Source: CAD feature listing. Evaluate the final solid. Frame: model axes, mm. A direction names the side the tool comes from. Coordinates: 2 decimals unless noted, no trailing zeros. Order: outer loops, then holes, each group sorted by start corner. A loop starts at its lowest first (then second) coordinate and runs counter-clockwise, first axis right, second up. Notation, with made-up numbers: (8, -13) -> (67, -13) arc R16 cw to (67, -2) -> close; hole circle Ø9 at (74.25, -17). An arc over 180 degrees is marked (long way). Write item = value, one per line. Start each with the question number.
Item 1: Section query C-C (y = 9). Output: boundary loops of the cut face in (x, z).
Item 2: Contact query for flat-ended pins moving along their axis: pin 1 (2 mm diameter, centred on x = 24.5, y = -39, fed in from +Z); pin 2 (5 mm diameter, centred on x = 26, z = -12.5, fed in from -Y); pin 3 (12 mm diameter, centred on y = 19.5, z = -18, fed in from -X). Output: stop coordinate, or through.
Item 3: Ray query, line 1 along Z through (x, y) = (16.25, 26.5); line 2 along Y through (x, z) = (28.75, -15); line 3 along Y through (x, z) = (21.75, -2). Return the intervals inside material, ascending. Write a range as [from, to].
Item 4: Mould query, pull axis Z, two halves, no side actions, for faces 4 (the flat face through (26.737, 26, 0)), 5 (the flat face through (26, 23, -2.473)), 6 (the flat face through (25.094, -47.195, 0.467)), 7 (the flat face through (25.02, -47.19, 1.6)). Classes: released by +Z, released by -Z, zero draft, split by the parting line, or undercut.
Item 5: Set-up query: faces 1 (the flat face through (28.04, -47.19, 1.47)), 2 (the flat face through (26.54, -47.34, -10.64)), 3 (the flat face through (26, 23, 2.253)). Return all of +Z, -Z, +X, -X, +Y, -Y with unobstructed straight access to the full face (end or side cutting, diameter ignored); none if empty.
Item 6: Section query B-B (z = 21). Output: boundary loops of the cut face in (x, y), then the cut area to 3 significant figures.
Item 7: Section query D-D (x = 30). Output: boundary loops of the cut face in (y, z), then the cut area to 3 significant figures.
Item 8: Section query A-A (z = -14.5). Output: boundary loops of the cut face in (x, y), then the cut area to 3 significant figures.
```python
from build123d import *

# Parameters (mm, degrees)
BOSS_EXTRUDE1_DEPTH  = 20
BOSS_EXTRUDE2_DEPTH  = 60
SKETCH3_R            = 10
BOSS_EXTRUDE3_DEPTH  = 12
SKETCH6_R            = 1.5
BOSS_EXTRUDE4_DEPTH  = 3
SKETCH7_W            = 45.133553402
SKETCH7_H            = 10.461726886
BOSS_EXTRUDE5_DEPTH  = 4
SKETCH9_W            = 2
SKETCH9_H            = 10.461726886
CUT_EXTRUDE2_DEPTH   = 22
SKETCH10_W           = 2
SKETCH10_H           = 10.461726886
CUT_EXTRUDE3_DEPTH   = 22
CUT_EXTRUDE7_DEPTH   = 60
CUT_EXTRUDE8_DEPTH   = 60
SKETCH20_W           = 0.930986134
SKETCH20_H           = 37.401550855
CUT_EXTRUDE9_DEPTH   = 7
SKETCH21_W           = 7
SKETCH21_H           = 37.143096713
CUT_EXTRUDE10_DEPTH  = 7
SKETCH24_W           = 7
SKETCH24_H           = 37.288200147
CUT_EXTRUDE11_DEPTH  = 7
SKETCH25_W           = 0.930986134
SKETCH25_H           = 37.288200147
CUT_EXTRUDE12_DEPTH  = 7
SKETCH31_W           = 2.173787646
SKETCH31_H           = 4.725625318
BOSS_EXTRUDE8_DEPTH  = 12
SKETCH32_R           = 7.5
BOSS_EXTRUDE12_DEPTH = 5
SKETCH35_R           = 7.5
BOSS_EXTRUDE14_DEPTH = 8


with BuildPart() as part:
    # Sketch1 → Boss-Extrude1 (new body)
    with BuildSketch(Plane(origin=(0, 0, 0), x_dir=(1, 0, 0), z_dir=(0, 1, 0))):
        with BuildLine():
            Line((24.096630412, 22.546671656), (22.159303529, -24.453328344))
            ThreePointArc((22.159303529, -24.453328344), (32.972001095, -1.359096683), (24.096630412, 22.546671656))
        make_face()
    extrude(amount=BOSS_EXTRUDE1_DEPTH)

    # Sketch2 → Boss-Extrude2 (add)
    with BuildSketch(Plane.XZ):
        with BuildLine():
            Line((22.159303529, 24.453328344), (24.096630412, -22.546671656))
            ThreePointArc((24.096630412, -22.546671656), (24.546704066, -22.055822802), (24.986780993, -21.55599164))
            Line((24.986780993, -21.55599164), (23.127966971, 23.539268124))
            ThreePointArc((23.127966971, 23.539268124), (22.648247037, 24.001185515), (22.159303529, 24.453328344))
        make_face()
    extrude(amount=BOSS_EXTRUDE2_DEPTH)

    # Sketch3 → Boss-Extrude3 (add)
    with BuildSketch(Plane(origin=(23.127966971, 0, 0.953328344), x_dir=(-0.041184748, 0, 0.999151548), z_dir=(-0.999151548, 0, -0.041184748))):
        with Locations((0, -47)):
            Circle(SKETCH3_R)
    extrude(amount=BOSS_EXTRUDE3_DEPTH)

    # Sketch6 → Boss-Extrude4 (add)
    with BuildSketch(Plane(origin=(24.057373982, 0, 0.991638242), x_dir=(0.041184748, 0, -0.999151548), z_dir=(0.999151548, 0, 0.041184748))):
        with Locations((0, -47)):
            Circle(SKETCH6_R)
    extrude(amount=BOSS_EXTRUDE4_DEPTH)

    # Sketch7 → Boss-Extrude5 (add)
    with BuildSketch(Plane(origin=(24.057373982, 0, 0.991638242), x_dir=(0.041184748, 0, -0.999151548), z_dir=(0.999151548, 0, 0.041184748))):
        with Locations((0, -47.268051565)):
            Rectangle(SKETCH7_W, SKETCH7_H)
    extrude(amount=BOSS_EXTRUDE5_DEPTH)

    # Sketch9 → Cut-Extrude2 (cut)
    with BuildSketch(Plane(origin=(-0.929407011, 0, 22.547629882), x_dir=(0.999151548, 0, 0.041184748), z_dir=(-0.041184748, 0, 0.999151548))):
        with Locations((25.077802834, -47.268051565)):
            Rectangle(SKETCH9_W, SKETCH9_H)
    extrude(amount=-CUT_EXTRUDE2_DEPTH, mode=Mode.SUBTRACT)

    # Sketch10 → Cut-Extrude3 (cut)
    with BuildSketch(Plane(origin=(0.929407011, 0, -22.547629882), x_dir=(-0.999151548, 0, -0.041184748), z_dir=(0.041184748, 0, -0.999151548))):
        with Locations((-25.077802834, -47.268051565)):
            Rectangle(SKETCH10_W, SKETCH10_H)
    extrude(amount=-CUT_EXTRUDE3_DEPTH, mode=Mode.SUBTRACT)

    # Sketch16 → Cut-Extrude7 (cut)
    with BuildSketch(Plane.XZ.offset(60)):
        with BuildLine():
            Line((22.159303529, 24.453328344), (22.688611434, 11.612195682))
            Line((22.688611434, 11.612195682), (23.619597568, 11.612195682))
            Line((23.619597568, 11.612195682), (23.127966971, 23.539268124))
            ThreePointArc((23.127966971, 23.539268124), (22.648247037, 24.001185515), (22.159303529, 24.453328344))
        make_face()
    extrude(amount=-CUT_EXTRUDE7_DEPTH, mode=Mode.SUBTRACT)

    # Sketch19 → Cut-Extrude8 (cut)
    with BuildSketch(Plane.XZ.offset(60)):
        with BuildLine():
            Line((23.571126961, -9.797835906), (24.502113095, -9.797835906))
            Line((24.502113095, -9.797835906), (24.986780993, -21.55599164))
            ThreePointArc((24.986780993, -21.55599164), (24.546704066, -22.055822802), (24.096630412, -22.546671656))
            Line((24.096630412, -22.546671656), (23.571126961, -9.797835906))
        make_face()
    extrude(amount=-CUT_EXTRUDE8_DEPTH, mode=Mode.SUBTRACT)

    # Sketch20 → Cut-Extrude9 (cut)
    with BuildSketch(Plane(origin=(0, 0, -9.797835906), x_dir=(-1, 0, 0), z_dir=(0, 0, -1))):
        with Locations((-24.036620028, -18.700775428)):
            Rectangle(SKETCH20_W, SKETCH20_H)
    extrude(amount=-CUT_EXTRUDE9_DEPTH, mode=Mode.SUBTRACT)

    # Sketch21 → Cut-Extrude10 (cut)
    with BuildSketch(Plane(origin=(23.571126961, 0, 0), x_dir=(0, 0, -1), z_dir=(1, 0, 0))):
        with Locations((6.297835906, -18.571548357)):
            Rectangle(SKETCH21_W, SKETCH21_H)
    extrude(amount=-CUT_EXTRUDE10_DEPTH, mode=Mode.SUBTRACT)

    # Sketch24 → Cut-Extrude11 (cut)
    with BuildSketch(Plane(origin=(24.057373982, 0, 0.991638242), x_dir=(0.041184748, 0, -0.999151548), z_dir=(0.999151548, 0, 0.041184748))):
        with Locations((-7.129576122, -18.644100074)):
            Rectangle(SKETCH24_W, SKETCH24_H)
    extrude(amount=-CUT_EXTRUDE11_DEPTH, mode=Mode.SUBTRACT)

    # Sketch25 → Cut-Extrude12 (cut)
    with BuildSketch(Plane.XY.offset(11.612195682)):
        with Locations((23.154104501, -18.644100074)):
            Rectangle(SKETCH25_W, SKETCH25_H)
    extrude(amount=-CUT_EXTRUDE12_DEPTH, mode=Mode.SUBTRACT)

    # Sketch31 → Boss-Extrude8 (add)
    with BuildSketch(Plane(origin=(0, 20, 0), x_dir=(1, 0, 0), z_dir=(0, 1, 0))):
        with Locations((25.650353258, 0.109937353)):
            Rectangle(SKETCH31_W, SKETCH31_H)
    extrude(amount=BOSS_EXTRUDE8_DEPTH)

    # Sketch32 → Boss-Extrude12 (add)
    with BuildSketch(Plane.XY.offset(2.252875306)):
        with Locations((19.150620534, 29.860210164)):
            Circle(SKETCH32_R)
    extrude(amount=BOSS_EXTRUDE12_DEPTH)

    # Sketch35 → Boss-Extrude14 (add)
    with BuildSketch(Plane(origin=(0, 0, 2.252875306), x_dir=(-1, 0, 0), z_dir=(0, 0, -1))):
        with Locations((-19.150620534, 29.860210164)):
            Circle(SKETCH35_R)
    extrude(amount=BOSS_EXTRUDE14_DEPTH)


solid = part.part
```
Computed:
q1.outline = (22.16, 24.45) -> (24.1, -22.55) arc R33 ccw to start
q2.pin_1 = 11.61
q2.pin_2 = -52.5
q2.pin_3 = 23.66
q3.line_1 = [-5.75, 7.25]
q3.line_2 = [0, 20]
q3.line_3 = [-56.57, -37.43], [22.83, 36.9]
q4.face_4 = zero draft
q4.face_5 = released by -Z
q4.face_6 = undercut
q4.face_7 = undercut
q5.face_1 = +Z, +X, -Y
q5.face_2 = -Z, -Y
q5.face_3 = +Z, +X
q6.outline = (22.3, 0) -> (25.46, 0) -> (25.46, 20) -> (22.3, 20) -> close; (25.23, -52.5) -> (27.24, -52.5) -> (27.24, -42.04) -> (25.23, -42.04) -> close
q6.area = 84.0 mm^2
q7.outline = (0, -13.75) -> (20, -13.75) -> (20, 13.75) -> (0, 13.75) -> close
q7.area = 550 mm^2
q8.outline = (23.76, 0) -> (29.64, 0) -> (29.64, 20) -> (23.76, 20) -> close; (26.7, -52.5) -> (28.7, -52.5) -> (28.7, -42.04) -> (26.7, -42.04) -> close
q8.area = 139 mm^2
